The model under review builds one solid part; all positions refer to its coordinate system, in mm. Give positions to 0.01 mm unless a question says otherwise; leave off trailing zeros. Order: outer loops, then holes, each group sorted by start corner. A loop starts at its lowest first (then second) coordinate and runs counter-clockwise, first axis right, second up. Notation, with made-up numbers: (36, 12) -> (58, 12) arc R12 ccw to (58, 22) -> close; hole circle Ø3 at (48.5, 71.25). An arc over 180 degrees is marked (long way). Answer as a JSON object with one key per item and string values. Group by question number.
Autodesk Inventor part; units mm, degrees
ref_plane "YZ Plane" through (0, 0, 0) normal (1, 0, 0) x (0, 1, 0)
ref_plane "XZ Plane" through (0, 0, 0) normal (0, 1, 0) x (-1, 0, 0)
ref_plane "XY Plane" through (0, 0, 0) normal (0, 0, 1) x (1, 0, 0)
sketch "Sketch1" plane through (0, 0, 0) normal (0, 1, 0) x (-1, 0, 0)
  circle A0 centre (0, 0) radius 9.25
  circle A1 centre (0, 0) radius 13.75 construction
  circle A2 centre (9.7227, -9.7227) radius 1.7
  line L0 (9.7227, -9.7227) -> (0, 0) construction
  circle A3 centre (9.7227, 9.7227) radius 1.7
  circle A4 centre (-9.7227, 9.7227) radius 1.7
  circle A5 centre (-9.7227, -9.7227) radius 1.7
  line L1 (0, 0) -> (0, -13.75) construction
  circle A6 centre (0, 0) radius 17.5
  circle A7 centre (0, 0) radius 10 construction
  line L2 (5, 16.7705) -> (0, 13.75) construction
  line L3 (0, 13.75) -> (-5, 16.7705) construction
  spline S0 degree 2 poles (5, 16.7705) (0, 13.75) (-5, 16.7705) knots 1 1 1 2 2 2
  line L4 (5, 16.7705) -> (-5, 16.7705) construction
  line L5 (0, 13.75) -> (0, 10) construction
  dimension "d10" = 20
  dimension "d0" = 18.5
  dimension "d2" = 3.4
  dimension "d6" = 360
  dimension "d8" = 45
  dimension "d11" = 10
  dimension "d30" = 7.5
  dimension "d31" = 3.75
extrude "Extrusion1" add sketch "Sketch1" along normal blind 5 contours A2 | A3 | A4 | A5 | A6 S0 picked at (12.2147, -4.9313)
fillet "Fillet1" radius 2 2 edges at (-5, 2.5, 16.7705) (5, 2.5, 16.7705)
chamfer "Chamfer1" distance 0.5 angle 45 2 edges at (9.25, 5, 0) (9.25, 0, 0)
chamfer "Chamfer2" distance 0.5 angle 45 8 edges at (0, 5, -17.5) (-5.0769, 5, 16.5928) (0, 5, 15.2603) (5.0769, 5, 16.5928) (0, 0, -17.5) (-5.0769, 0, 16.5928) (0, 0, 15.2603) (5.0769, 0, 16.5928)
properties part number "Motor Mount" material "ABS Plastic"
1. Take a section at A-A on z = 0. Give the boundary of the cut face in (x, y), plus the area to 3 significant figures.
2. For probe 1 along Z at (x, y) = (0, 2.8); probe 2 along Z at (x, y) = (6, 2.7); probe 3 along X at (y, z) = (4.3, 5.5), list the stretches that pass through material, from the lowest coordinate up. Write a range as [from, to].
3. Draft analysis for pull direction X (two halves, no side actions). For faces 1 (the cylindrical face through (2.01, 2.47, 9.03)), 2 (the flat face through (-7.3, 5, 7.1)), 3 (the conical face through (0.671, 0.142, -17.129)), state which applies: pulls with the +X half, pulls with the -X half, needs draft (parallel to the pull), parting line crosses it, or undercut.
4. For pin 1 (1 mm diameter, centred on y = 2.5, z = -9, fed in from +X); pin 2 (10 mm diameter, centred on x = 12, z = 13, fed in from -Y); pin 3 (3 mm diameter, centred on x = -14, y = 2.5, fed in from +Z); pin 4 (1 mm diameter, centred on y = 1, z = -1.5, fed in from -X), all flat-tipped, find the tip position at first contact; note any pin that passes through.
Checks:
{
 "1": {"outline": "(-17.5, 0.5) -> (-17, 0) -> (-9.75, 0) -> (-9.25, 0.5) -> (-9.25, 4.5) -> (-9.75, 5) -> (-17, 5) -> (-17.5, 4.5) -> close; (9.25, 0.5) -> (9.75, 0) -> (17, 0) -> (17.5, 0.5) -> (17.5, 4.5) -> (17, 5) -> (9.75, 5) -> (9.25, 4.5) -> close", "area": "81.5 mm2"},
 "2": {"probe 1": "z = [-17.5, -9.25], [9.25, 15.26]", "probe 2": "z = [-16.44, -7.04], [7.04, 16.44]", "probe 3": "x = [-16.61, -7.44], [7.44, 16.61]"},
 "3": {"face 1": "undercut", "face 2": "needs draft", "face 3": "parting line crosses it"},
 "4": {"pin 1": "stops at x = 15.3", "pin 2": "stops at y = 0", "pin 3": "stops at z = 12.25", "pin 4": "stops at x = -17.47"}
}
